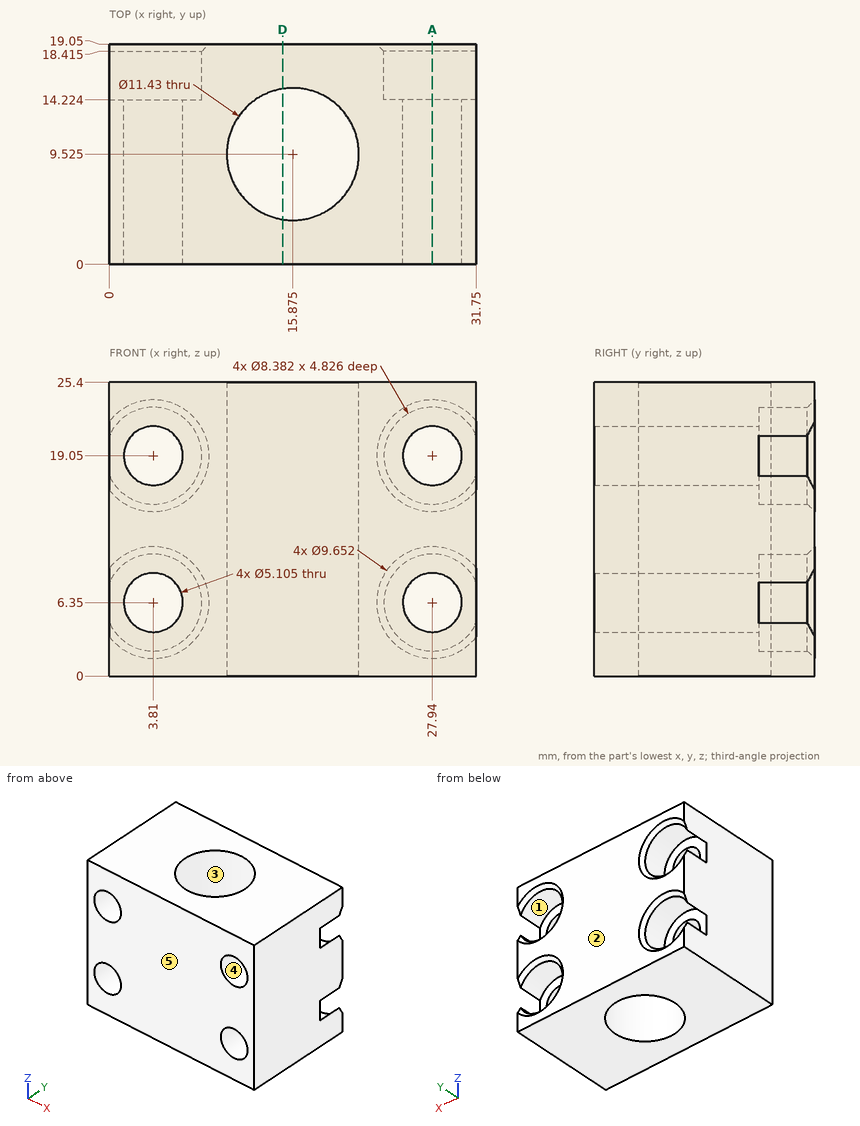
Geometry check sheet. Reference: drawing and pictorial views, mm from the part's lowest x, y, z. A direction names the side the tool comes from. Give positions to 0.01 mm unless a question says otherwise; leave off trailing zeros. Order: outer loops, then holes, each group sorted by start corner. A loop starts at its lowest first (then second) coordinate and runs counter-clockwise, first axis right, second up. Notation, with made-up numbers: M -4,49 L 19,49 A15 cw 19,75 Z; hole C -19,76.25 d4. An arc over 180 degrees is marked long. Answer in a Markdown table with one row per item.
1) Release check for a two-part mould opening along Y. For the marked faces 3, 4 and 5 record: +Y half, -Y half, draft (parallel to the pull), parting line (faces both ways), or undercut.
Filled sheet:
| item | result |
|---|---|
| face 3 | undercut |
| face 4 | draft |
| face 5 | -Y half |
2) Cross-section at A-A, the plane x = 27.94. Count the separate pieces of the cut face and the enclosed holes in it, plus the area to 3 significant figures.
Filled sheet:
| item | result |
|---|---|
| separate pieces | 3 |
| enclosed holes | 0 |
| area | 257 mm2 |
3) Cross-section at D-D, the plane x = 15. Enter the section's corners in (y, z), plus the area to 3 significant figures.
Filled sheet:
| item | result |
|---|---|
| outline | M 0,0 L 3.88,0 L 3.88,25.4 L 0,25.4 Z; M 15.17,0 L 19.05,0 L 19.05,25.4 L 15.17,25.4 Z |
| area | 197 mm2 |
4) Thickness scan on L1, parallel to Z at x = 28, y = 16.5; L2, parallel to X at y = 11.25, z = 19.05; L3, parallel to Y at x = 7.5, z = 19. Record the ranges inside material, lowest first. Write a range as [from, to].
Filled sheet:
| item | result |
|---|---|
| L1 | z = [0, 2.16], [10.54, 14.86], [23.24, 25.4] |
| L2 | x = [0, 1.26], [6.36, 10.43], [21.32, 25.39], [30.49, 31.75] |
| L3 | y = [0, 14.22] |
5) Access from +Z, -Z, +X, -X, +Y, -Y to the whole of each face (thin tool, end or side, straight path). Record for the marked faces 1 and 2.
Filled sheet:
| item | result |
|---|---|
| face 1 | +Y |
| face 2 | +Z, -Z, +X, -X, +Y |
6) Gauge pin test, flat ends, axial feed: P1, Ø6.5, axis at x = 3.81, z = 19.05, coming from the +Y side; P2, Ø6.5, axis at x = 29.5, z = 19.5, coming from the +Y side. Record the tip position at first contact, or that the pin passes through.
Filled sheet:
| item | result |
|---|---|
| P1 | stops at y = 14.22 |
| P2 | stops at y = 18.95 |
